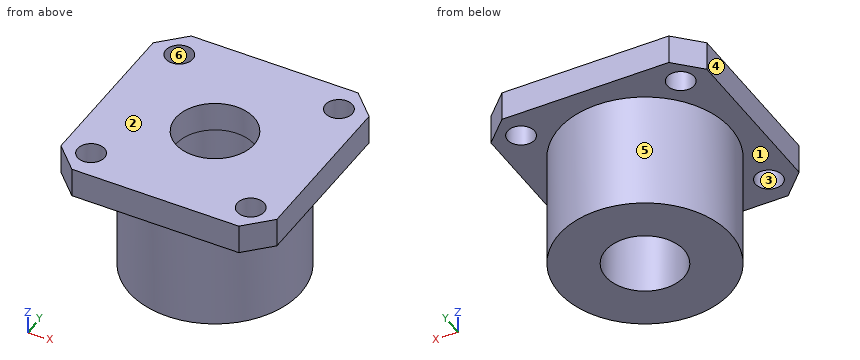
from build123d import *

# Parameters (mm, degrees)
SKETCH_1_W          = 44
SKETCH_1_H          = 44
SKETCH_1_R          = 2.75
EXTRUDE_1_DEPTH     = 6
CHAMFER_1_SIZE      = 5
SKETCH_2_R          = 17.5
SKETCH_2_R_2        = 8
EXTRUDE_2_DEPTH     = 24
SKETCH_3_R          = 8
CUT_EXTRUDE_1_DEPTH = 40.293765409


with BuildPart() as part:
    # 草图1 → 凸台-拉伸1 (new body)
    with BuildSketch(Plane.XY):
        Rectangle(SKETCH_1_W, SKETCH_1_H)
        with Locations((-16.263455967, 16.263455967)):
            Circle(SKETCH_1_R, mode=Mode.SUBTRACT)
        with Locations((16.263455967, 16.263455967)):
            Circle(SKETCH_1_R, mode=Mode.SUBTRACT)
        with Locations((16.263455967, -16.263455967)):
            Circle(SKETCH_1_R, mode=Mode.SUBTRACT)
        with Locations((-16.263455967, -16.263455967)):
            Circle(SKETCH_1_R, mode=Mode.SUBTRACT)
    extrude(amount=EXTRUDE_1_DEPTH)

    # 倒角1
    chamfer_1_edges = [part.edges().sort_by_distance(p)[0] for p in [
        (-22, 22, 3),
        (22, 22, 3),
        (22, -22, 3),
        (-22, -22, 3),
    ]]
    chamfer(chamfer_1_edges, length=CHAMFER_1_SIZE)

    # 草图2 → 凸台-拉伸2 (add)
    with BuildSketch(Plane(origin=(0, 0, 0), x_dir=(-1, 0, 0), z_dir=(0, 0, -1))):
        with Locations(Location((0, 0, 0), (0, 0, 180))):
            Circle(SKETCH_2_R)
        Circle(SKETCH_2_R_2, mode=Mode.SUBTRACT)
    extrude(amount=EXTRUDE_2_DEPTH)

    # 草图3 → 切除-拉伸1 (cut, through all)
    with BuildSketch(Plane(origin=(0, 0, 0), x_dir=(-1, 0, 0), z_dir=(0, 0, -1))):
        Circle(SKETCH_3_R)
    extrude(amount=-CUT_EXTRUDE_1_DEPTH, mode=Mode.SUBTRACT)


solid = part.part
Check sheet for the modelled part. Datum: model origin and axes. Units: mm. Face numbers are marked on the shaded views. A direction names the side the tool comes from. Give positions to 0.01 mm unless a question says otherwise; leave off trailing zeros. Write each loop counter-clockwise with the first axis right and the second up, starting at its lowest first coordinate (ties: lowest second). Pieces come first, ordered by that corner, then holes. Notation, with made-up numbers: (70, -24) -> (124, -24) arc R19 ccw to (124, 4) -> close; hole circle Ø8 at (44.25, 18). An arc over 180 degrees is marked (long way). Use one line per item in the form item = value. Start each with the question number.
1. Mould release check, pull along Y, two halves, no side actions. Record for the marked faces 3, 4, 5 and 6: pulls with the +Y half, pulls with the -Y half, needs draft (parallel to the pull), parting line crosses it, or undercut.
2. Section check C-C (z = 1.75). Record the cut outline in (x, y).
3. Go/stop test with flat-tipped pins: P1, Ø2, axis at x = 14, y = 16.5, coming from the -Z side; P2, Ø4, axis at y = 14.5, z = -8, coming from the +X side; P3, Ø2, axis at x = 14.5, z = -12, coming from the -Y side. Record where each tip stops, or that it passes through.
4. Section check D-D (x = -12.5). Record the cut outline in (y, z), and give its area (3 significant figures).
5. Access from +Z, -Z, +X, -X, +Y, -Y to the whole of each face (thin tool, end or side, straight path). Record for the marked faces 1 and 2.
6. Thickness scan on line 1 along Y through (x, z) = (0, 3.35); line 2 along Y through (x, z) = (18, 0.5); line 3 along Y through (x, z) = (0, -11.25). Record the ranges inside material, lowest first. Write a range as from..to.
7. Section check A-A (x = 0). Record the cut outline in (y, z), and give its area (3 significant figures).
Conclusion:
q1.face_3 = undercut
q1.face_4 = needs draft
q1.face_5 = parting line crosses it
q1.face_6 = undercut
q2.outline = (-22, -17) -> (-17, -22) -> (17, -22) -> (22, -17) -> (22, 17) -> (17, 22) -> (-17, 22) -> (-22, 17) -> close; hole circle Ø5.5 at (-16.26, -16.26); hole circle Ø5.5 at (-16.26, 16.26); hole circle Ø16 at (0, 0); hole circle Ø5.5 at (16.26, -16.26); hole circle Ø5.5 at (16.26, 16.26)
q3.P1 = 0
q3.P2 = 12.25
q3.P3 = -11.14
q4.outline = (-22, 0) -> (-12.25, 0) -> (-12.25, -24) -> (12.25, -24) -> (12.25, 0) -> (22, 0) -> (22, 6) -> (-22, 6) -> close
q4.area = 852 mm²
q5.face_1 = -Z
q5.face_2 = +Z, +X, -X, +Y, -Y
q6.line_1 = -22..-8, 8..22
q6.line_2 = -21..-18.4, -14.13..14.13, 18.4..21
q6.line_3 = -17.5..-8, 8..17.5
q7.outline = (-22, 0) -> (-17.5, 0) -> (-17.5, -24) -> (-8, -24) -> (-8, 6) -> (-22, 6) -> close; (8, -24) -> (17.5, -24) -> (17.5, 0) -> (22, 0) -> (22, 6) -> (8, 6) -> close
q7.area = 624 mm²
